For this review, take the finished solid that the model builds, in its own axes (mm). Coordinates: 2 decimals unless noted, no trailing zeros. Write each loop counter-clockwise with the first axis right and the second up, starting at its lowest first coordinate (ties: lowest second). Pieces come first, ordered by that corner, then holes.
1) We need section C-C on z = -16.5. Write out the cut boundary in (x, y), then the cut area to 3 significant figures.
2) We need section A-A on x = 10. Write out the cut boundary in (y, z), then the cut area to 3 significant figures.
3) Mouldability with a two-part tool opening along Y and no side actions: class faces 1 (the face through (0, 10, 0)), 2 (the face through (11.686, 1.909, -1.075)), 3 (the face through (11.908, 5.601, -9.86)) as pulls with the +Y half, pulls with the -Y half, needs draft (parallel to the pull), parting line crosses it, or undercut.
4) We need section B-B on y = 1. Write out the cut boundary in (x, z), then the cut area to 3 significant figures.
5) To check wall thickness, follow line 1 along X through (y, z) = (5, 11.75); line 2 along Y through (x, z) = (-10, 7.5); line 3 along Z through (x, y) = (10, 7.8). State the ranges of each line that lie inside material, in increasing order.
6) Insertion check: P1, Ø4.5, axis at x = 10, z = 0, coming from the +Y side. The pin has a flat end and moves straight along its axis. Give the tip position at first contact, or say it passes through.
from build123d import *

# Parameters (mm, degrees)
SKETCH2_W           = 40
SKETCH2_H           = 40
BOSS_EXTRUDE1_DEPTH = 10
SKETCH3_R           = 2
CUT_EXTRUDE1_DEPTH  = 51
SKETCH4_R           = 2
CUT_EXTRUDE2_DEPTH  = 12


with BuildPart() as part:
    # Sketch2 → Boss-Extrude1 (new body)
    with BuildSketch(Plane(origin=(0, 0, 0), x_dir=(1, 0, 0), z_dir=(0, 1, 0))):
        Rectangle(SKETCH2_W, SKETCH2_H)
    extrude(amount=BOSS_EXTRUDE1_DEPTH)

    # Sketch3 → Cut-Extrude1 (cut)
    with BuildSketch(Plane.XY.offset(20)):
        with Locations((10, 5)):
            Circle(SKETCH3_R)
        with Locations((-10, 5)):
            Circle(SKETCH3_R)
    extrude(amount=-CUT_EXTRUDE1_DEPTH, mode=Mode.SUBTRACT)

    # Sketch4 → Cut-Extrude2 (cut)
    with BuildSketch(Plane.XZ):
        with Locations(Location((10, 0, 0), (0, 0, 270))):
            Circle(SKETCH4_R)
        with Locations(Location((-10, 0, 0), (0, 0, 270))):
            Circle(SKETCH4_R)
    extrude(amount=-CUT_EXTRUDE2_DEPTH, mode=Mode.SUBTRACT)


solid = part.part
Result:
1. outline: (-20, 0) - (20, 0) - (20, 10) - (-20, 10) - close; hole circle Ø4 at (-10, 5); hole circle Ø4 at (10, 5)
1. area: 375 mm2
2. outline: (0, -20) - (3, -20) - (3, -2) - (0, -2) - close; (0, 2) - (3, 2) - (3, 20) - (0, 20) - close; (7, -20) - (10, -20) - (10, -2) - (7, -2) - close; (7, 2) - (10, 2) - (10, 20) - (7, 20) - close
2. area: 216 mm2
3. face 1: pulls with the +Y half
3. face 2: needs draft
3. face 3: undercut
4. outline: (-20, -20) - (20, -20) - (20, 20) - (-20, 20) - close; hole circle Ø4 at (-10, 0); hole circle Ø4 at (10, 0)
4. area: 1,570 mm2
5. line 1: x = -20 to -12, -8 to 8, 12 to 20
5. line 2: y = 0 to 3, 7 to 10
5. line 3: z = -20 to -2, 2 to 20
6. P1: stops at y = 10
